```python
from build123d import *

# Parameters (mm, degrees)
F0_R     = 6.35
F1_DEPTH = 38.1
F2_DEPTH = 25.4
F3_DEPTH = 12.7


with BuildPart() as f1:
    # F0 (on Top) → F1 (new body)
    with BuildSketch(Plane.XY):
        with BuildLine():
            ThreePointArc((-63.5, -31.75), (-61.6401280605, -36.2401280605), (-57.15, -38.1))
            Line((-57.15, -38.1), (57.15, -38.1))
            ThreePointArc((57.15, -38.1), (61.6401280605, -36.2401280605), (63.5, -31.75))
            Line((63.5, -31.75), (63.5, 31.75))
            ThreePointArc((63.5, 31.75), (61.6401280605, 36.2401280605), (57.15, 38.1))
            Line((57.15, 38.1), (-57.15, 38.1))
            ThreePointArc((-57.15, 38.1), (-61.6401280605, 36.2401280605), (-63.5, 31.75))
            Line((-63.5, 31.75), (-63.5, -31.75))
        make_face()
        with BuildLine():
            ThreePointArc((-57.15, 25.4), (-55.2901280605, 29.8901280605), (-50.8, 31.75))
            Line((-50.8, 31.75), (50.8, 31.75))
            ThreePointArc((50.8, 31.75), (55.2901280605, 29.8901280605), (57.15, 25.4))
            Line((57.15, 25.4), (57.15, -25.4))
            ThreePointArc((57.15, -25.4), (55.2901280605, -29.8901280605), (50.8, -31.75))
            Line((50.8, -31.75), (-50.8, -31.75))
            ThreePointArc((-50.8, -31.75), (-55.2901280605, -29.8901280605), (-57.15, -25.4))
            Line((-57.15, -25.4), (-57.15, 25.4))
        make_face(mode=Mode.SUBTRACT)
        with BuildLine():
            Line((50.8, 31.75), (-50.8, 31.75))
            ThreePointArc((-50.8, 31.75), (-55.2901280605, 29.8901280605), (-57.15, 25.4))
            Line((-57.15, 25.4), (-57.15, -25.4))
            ThreePointArc((-57.15, -25.4), (-55.2901280605, -29.8901280605), (-50.8, -31.75))
            Line((-50.8, -31.75), (50.8, -31.75))
            ThreePointArc((50.8, -31.75), (55.2901280605, -29.8901280605), (57.15, -25.4))
            Line((57.15, -25.4), (57.15, 25.4))
            ThreePointArc((57.15, 25.4), (55.2901280605, 29.8901280605), (50.8, 31.75))
        make_face()
        with BuildLine():
            Line((-57.15, 57.15), (-57.15, 38.1))
            Line((-57.15, 38.1), (57.15, 38.1))
            Line((57.15, 38.1), (57.15, 57.15))
            ThreePointArc((57.15, 57.15), (55.2901280605, 61.6401280605), (50.8, 63.5))
            Line((50.8, 63.5), (-50.8, 63.5))
            ThreePointArc((-50.8, 63.5), (-55.2901280605, 61.6401280605), (-57.15, 57.15))
        make_face()
        with Locations((-26.5334639698, 50.8)):
            Circle(F0_R, mode=Mode.SUBTRACT)
        with Locations((-1.1334639698, 50.8)):
            Circle(F0_R, mode=Mode.SUBTRACT)
        with Locations((24.2665360302, 50.8)):
            Circle(F0_R, mode=Mode.SUBTRACT)
        with Locations((-26.5334639698, 50.8)):
            Circle(F0_R)
        with Locations((-1.1334639698, 50.8)):
            Circle(F0_R)
        with Locations((24.2665360302, 50.8)):
            Circle(F0_R)
    extrude(amount=-F1_DEPTH)

    # F0 (on Top) → F2 (cut)
    with BuildSketch(Plane.XY):
        with BuildLine():
            Line((50.8, 31.75), (-50.8, 31.75))
            ThreePointArc((-50.8, 31.75), (-55.2901280605, 29.8901280605), (-57.15, 25.4))
            Line((-57.15, 25.4), (-57.15, -25.4))
            ThreePointArc((-57.15, -25.4), (-55.2901280605, -29.8901280605), (-50.8, -31.75))
            Line((-50.8, -31.75), (50.8, -31.75))
            ThreePointArc((50.8, -31.75), (55.2901280605, -29.8901280605), (57.15, -25.4))
            Line((57.15, -25.4), (57.15, 25.4))
            ThreePointArc((57.15, 25.4), (55.2901280605, 29.8901280605), (50.8, 31.75))
        make_face()
    extrude(amount=-F2_DEPTH, mode=Mode.SUBTRACT)

    # F0 (on Top) → F3 (cut)
    with BuildSketch(Plane.XY):
        with Locations((-26.5334639698, 50.8)):
            Circle(F0_R)
        with Locations((-1.1334639698, 50.8)):
            Circle(F0_R)
        with Locations((24.2665360302, 50.8)):
            Circle(F0_R)
    extrude(amount=-F3_DEPTH, mode=Mode.SUBTRACT)


solid = f1.part
```
Here's how the part is built. I have some questions about the finished solid (model axes, mm). A direction names the side the tool comes from. Coordinates: 2 decimals unless noted, no trailing zeros. Write each loop counter-clockwise with the first axis right and the second up, starting at its lowest first coordinate (ties: lowest second). Pieces come first, ordered by that corner, then holes. Notation, with made-up numbers: M 41,75.25 L 93,75.25 A35 ccw 93,107.25 Z; hole C -35.5,-37 d10. An arc over 180 degrees is marked long. Answer as CSV lines item,"result". Start each with the question number.
Q1. Suppose I cut it at A-A, the plane y = 8. List the corners of the cut face in (x, z) for me, then the cut area to 3 significant figures.
Q2. Suppose I cut it at B-B, the plane z = -18. List the corners of the cut face in (x, y) for me.
Q3. Will these pins go through, and if not, where does the flat tip stop? pin 1 Ø2 at (y, z) = (46.5, -16) entering from -X; pin 2 Ø3 at (y, z) = (37, -24) entering from -X; pin 3 Ø4 at (x, y) = (-27.5, 52) entering from +Z.
Q4. If we mould it in two halves opening along Y, with no side actions, what happens to faces 1 (the cylindrical face through (-55.24, 61.69, -18.78)), 2 (the cylindrical face through (-1.96, 57.096, -6.261)), 3 (the cylindrical face through (-61.69, -36.19, -18.78))? For each: pulls with the +Y half, pulls with the -Y half, needs draft (parallel to the pull), parting line crosses it, or undercut.
Q5. For faces 4 (the flat face through (-1, 13, -38.1)), 5 (the flat face through (-1, 51, -12.7)), 6 (the flat face through (57.15, 47, -19)), which set-ups out of +Z, -Z, +X, -X, +Y, -Y let a thin tool reach every point of the face, with its end or its side?
Q6. Suppose I cut it at C-C, the plane x = -38. List the corners of the cut face in (y, z) for me, then the cut area to 3 significant figures.
Q7. I need wall thicknesses on probe 1 along Y at (x, z) = (24.5, -13.5); probe 2 along X at (y, z) = (-3, -10.5); probe 3 along X at (y, z) = (50, -9). Which ranges of each line are inside material? Lowest first, please. Write a range as [from, to].
Q8. Suppose I cut it at D-D, the plane z = -34. List the corners of the cut face in (x, y) for me, then the cut area to 3 significant figures.
Entries:
1,outline,"M -63.5,-38.1 L 63.5,-38.1 L 63.5,0 L 57.15,0 L 57.15,-25.4 L -57.15,-25.4 L -57.15,0 L -63.5,0 Z"
1,area,"1,940 mm²"
2,outline,"M -63.5,-31.75 A6.35 ccw -57.15,-38.1 L 57.15,-38.1 A6.35 ccw 63.5,-31.75 L 63.5,31.75 A6.35 ccw 57.15,38.1 L 57.15,57.15 A6.35 ccw 50.8,63.5 L -50.8,63.5 A6.35 ccw -57.15,57.15 L -57.15,38.1 A6.35 ccw -63.5,31.75 Z; hole M -57.15,-25.4 A6.35 ccw -50.8,-31.75 L 50.8,-31.75 A6.35 ccw 57.15,-25.4 L 57.15,25.4 A6.35 ccw 50.8,31.75 L -50.8,31.75 A6.35 ccw -57.15,25.4 Z"
3,pin 1,"stops at x = -57.15"
3,pin 2,"stops at x = -62.27"
3,pin 3,"stops at z = -12.7"
4,face 1,"pulls with the +Y half"
4,face 2,"undercut"
4,face 3,"pulls with the -Y half"
5,face 4,"-Z, +X, -X, +Y, -Y"
5,face 5,"+Z"
5,face 6,"+Z, -Z, +X, +Y"
6,outline,"M -38.1,-38.1 L 63.5,-38.1 L 63.5,0 L 31.75,0 L 31.75,-25.4 L -31.75,-25.4 L -31.75,0 L -38.1,0 Z"
6,area,"2,260 mm²"
7,probe 1,"y = [-38.1, -31.75], [31.75, 63.5]"
7,probe 2,"x = [-63.5, -57.15], [57.15, 63.5]"
7,probe 3,"x = [-57.15, -32.83], [-20.23, -7.43], [5.17, 17.97], [30.57, 57.15]"
8,outline,"M -63.5,-31.75 A6.35 ccw -57.15,-38.1 L 57.15,-38.1 A6.35 ccw 63.5,-31.75 L 63.5,31.75 A6.35 ccw 57.15,38.1 L 57.15,57.15 A6.35 ccw 50.8,63.5 L -50.8,63.5 A6.35 ccw -57.15,57.15 L -57.15,38.1 A6.35 ccw -63.5,31.75 Z"
8,area,"12,500 mm²"
